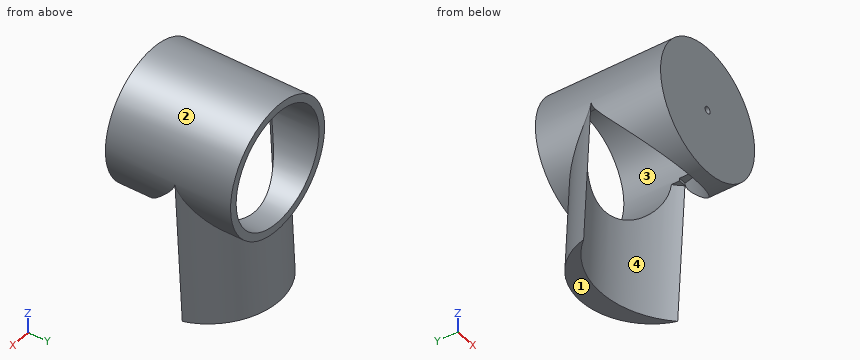
```python
from build123d import *
from build123d.topology import SkipClean

# Parameters (mm, degrees)
SKETCH1_R                        = 23.25
SKETCH1_R_2                      = 20.5
BOSS_EXTRUDE1_DEPTH              = 40
BOSS_EXTRUDE2_START              = -5
SKETCH1_2_R                      = 23.25
SKETCH1_2_R_2                    = 20.5
BOSS_EXTRUDE2_DEPTH              = 5
CUT_EXTRUDE1_DEPTH               = 35
BOSS_EXTRUDE3_REACH              = 88.878
BOSS_EXTRUDE3_END_RADIUS         = 23.25
CUT_EXTRUDE5_REACH               = 90.17
CUT_EXTRUDE5_OFFSET_FROM_SURFACE = 1
SKETCH5_R                        = 1.25
CUT_EXTRUDE6_DEPTH               = 10


with BuildPart() as part:
    # Sketch1 → Boss-Extrude1 (new body)
    with BuildSketch(Plane(origin=(0, 0, 0), x_dir=(1, 0, 0), z_dir=(0, 1, 0))):
        with Locations(Location((0, 0, 0), (0, 0, 270))):
            Circle(SKETCH1_R)
        with Locations(Location((0, 0, 0), (0, 0, 270))):
            Circle(SKETCH1_R_2, mode=Mode.SUBTRACT)
    extrude(amount=BOSS_EXTRUDE1_DEPTH)

    # Sketch1<2> → Boss-Extrude2 (add)
    # profile 1 of 2: a face of its own
    with BuildSketch(Plane(origin=(0, 0, 0), x_dir=(1, 0, 0), z_dir=(0, 1, 0)).offset(BOSS_EXTRUDE2_START)):
        with Locations(Location((0, 0, 0), (0, 0, 270))):
            Circle(SKETCH1_2_R)
        with Locations(Location((0, 0, 0), (0, 0, 270))):
            Circle(SKETCH1_2_R_2, mode=Mode.SUBTRACT)
    # profile 2 of 2: a face of its own
    with BuildSketch(Plane(origin=(0, 0, 0), x_dir=(1, 0, 0), z_dir=(0, 1, 0)).offset(BOSS_EXTRUDE2_START)):
        with Locations(Location((0, 0, 0), (0, 0, 270))):
            Circle(SKETCH1_2_R_2)
    extrude(amount=BOSS_EXTRUDE2_DEPTH)

    # Sketch2 → Cut-Extrude1 (cut)
    with BuildSketch(Plane.XY):
        with BuildLine():
            Line((23.25, 20), (-23.25, 20))
            ThreePointArc((-23.25, 20), (0, 0), (23.25, 20))
        make_face()
    extrude(amount=-CUT_EXTRUDE1_DEPTH, mode=Mode.SUBTRACT)

    # Boss-Extrude3: up to this cylinder (the profile starts outside it)
    with SkipClean():  # the faces are left unmerged after this step: merging them gives an invalid solid
        boss_extrude3_end = Plane(origin=(0, 34.101155, 0), z_dir=(0, -1, 0)) * Cylinder(BOSS_EXTRUDE3_END_RADIUS, 225.256, mode=Mode.PRIVATE)
        # Sketch3 → Boss-Extrude3 (add, up to the surface)
        with BuildSketch(Plane(origin=(0, 2.709163228, -51.693913872), x_dir=(1, 0, 0), z_dir=(0, -0.05233595624294392, 0.998629534754574)), mode=Mode.PRIVATE) as boss_extrude3_sk1:
            with BuildLine():
                ThreePointArc((-23.25, 19.972590695), (0, 30.650723957), (23.25, 19.972590695))
                ThreePointArc((23.25, 19.972590695), (0, 38.019650245), (-23.25, 19.972590695))
            make_face()
        boss_extrude3_tool1 = extrude(boss_extrude3_sk1.sketch, amount=BOSS_EXTRUDE3_REACH, mode=Mode.PRIVATE) - boss_extrude3_end
        add(boss_extrude3_tool1.solids().sort_by_distance((0, 34.101155, -50.048729))[0])

    # Cut-Extrude5: up to this face of the body (flat: up to its plane, moved by the offset)
    cut_extrude5_end = Plane(part.part.faces().sort_by_distance((-21.516068689, 17.104184879, 0))[0]).offset(CUT_EXTRUDE5_OFFSET_FROM_SURFACE)
    # Sketch4 → Cut-Extrude5 (cut, up to the picked face)
    with BuildSketch(Plane(origin=(0, 2.709163228, -51.693913872), x_dir=(1, 0, 0), z_dir=(0, -0.05233595624294392, 0.998629534754574)), mode=Mode.PRIVATE) as cut_extrude5_sk1:
        with BuildLine():
            ThreePointArc((23.25, 19.972590695), (0, 30.650723957), (-23.25, 19.972590695))
            add(Edge.make_bspline(
                [(-23.25, 19.972590695), (-23.25, 18.755779712), (0, 18.755779712), (23.25, 18.755779712), (23.25, 19.972590695)],
                knots=[3.141592654, 3.141592654, 3.141592654, 4.71238898, 4.71238898, 6.283185307, 6.283185307, 6.283185307], degree=2, weights=[1, 0.707106781, 1, 0.707106781, 1]))
        make_face()
    cut_extrude5_tool1 = split(extrude(cut_extrude5_sk1.sketch, amount=CUT_EXTRUDE5_REACH, mode=Mode.PRIVATE), bisect_by=cut_extrude5_end, keep=Keep.BOTH, mode=Mode.PRIVATE)
    add(cut_extrude5_tool1.solids().sort_by(Axis((0, 26.436495, -50.450417), (0, -0.05233595624294392, 0.998629534754574)))[0], mode=Mode.SUBTRACT)

    # Sketch5 → Cut-Extrude6 (cut)
    with BuildSketch(Plane(origin=(0, 0, 0), x_dir=(1, 0, 0), z_dir=(0, 1, 0))):
        with Locations(Location((0, 0, 0), (0, 0, 270))):
            Circle(SKETCH5_R)
    extrude(amount=-CUT_EXTRUDE6_DEPTH, mode=Mode.SUBTRACT)


solid = part.part
```
CAD build for the part. Positions are in the model's coordinates, mm. Face numbers are marked on the shaded views. A direction names the side the tool comes from. Give positions to 0.01 mm unless a question says otherwise; leave off trailing zeros. Order: outer loops, then holes, each group sorted by start corner. A loop starts at its lowest first (then second) coordinate and runs counter-clockwise, first axis right, second up. Notation, with made-up numbers: M -1.5,62.5 L 16.5,62.5 A20 cw 16.5,68.5 Z; hole C 73.25,4 d8. An arc over 180 degrees is marked long. Put each result on its own line as item: value. Start each with the question number.
(1) Saw through at A-A, the plane x = -12.5. Write the cut outline in (y, z).
(2) Drill centre lines: line 1 along X through (y, z) = (-1.9, 0); line 2 along X through (y, z) = (8, 0). Where is each one in solid material? Low to high.
(3) Saw through at B-B, the plane x = -5. Write the cut outline in (y, z).
(4) Flat gauge pins, fed straight in: pin 1 Ø20.5 at (x, z) = (-8.5, 3.5) entering from +Y; pin 2 Ø8 at (x, z) = (12.5, 11.5) entering from +Y; pin 3 Ø8 at (x, y) = (-4.5, 23.5) entering from +Z; pin 4 Ø12 at (y, z) = (0, -32) entering from -X. Where does each tip first touch, or does it go through?
(5) Which spindle directions (+Z, -Z, +X, -X, +Y, -Y) get a long thin tool onto all of the face, cutting with end or side? Do the marked faces 1, 2, 3 and 4. Say none if no direction does.
(6) Saw through at C-C, the plane y = 17. Write the cut outline in (x, z), then the cut area to 3 significant figures.
(7) Saw through at D-D, the plane z = -10. Give the number of separate pieces and of enclosed holes in the cut face, then the cut area to 3 significant figures.
Check result:
1. outline: M -5,-19.6 L 3.6,-19.6 L 3.6,-16.25 L 0,-16.25 L 0,16.25 L 40,16.25 L 40,19.6 L -5,19.6 Z; M 28.88,-16.25 L 30.66,-50.23 L 37.17,-49.89 L 35.58,-19.6 L 40,-19.6 L 40,-16.25 Z
2. line 1: x = -23.25 to -1.25, 1.25 to 23.25
2. line 2: x = -23.25 to -20.5, 20.5 to 23.25
3. outline: M -5,-22.71 L 0.54,-22.71 L 0.54,-19.88 L 0,-19.88 L 0,19.88 L 40,19.88 L 40,22.71 L -5,22.71 Z; M 31.32,-19.88 L 32.91,-50.11 L 40.15,-49.73 L 38.73,-22.71 L 40,-22.71 L 40,-19.88 Z
4. pin 1: stops at y = 0
4. pin 2: stops at y = 40
4. pin 3: stops at z = 23.24
4. pin 4: passes through
5. face 1: -Z, +X, -X, +Y
5. face 2: none
5. face 3: +Y
5. face 4: -Z
6. outline: M -22.59,-5.48 L -22.59,0 L -20.5,0 A20.5 cw 20.5,0 L 22.59,0 L 22.59,-5.48 A23.25 ccw long Z
6. area: 194 mm2
7. separate pieces: 3
7. enclosed holes: 0
7. area: 381 mm2
